The figure shows three views and two pictorial views of one solid part (mm, origin at its lowest corner). Answer the questions. A direction names the side the tool comes from. Coordinates: 2 decimals unless noted, no trailing zeros. Order: outer loops, then holes, each group sorted by start corner. A loop starts at its lowest first (then second) coordinate and runs counter-clockwise, first axis right, second up. Notation, with made-up numbers: (23.25, 66.5) -> (41.25, 66.5) arc R20 cw to (41.25, 93.5) -> close; hole circle Ø5 at (69.25, 56.25). An arc over 180 degrees is marked (long way). Write item = value, one per line.
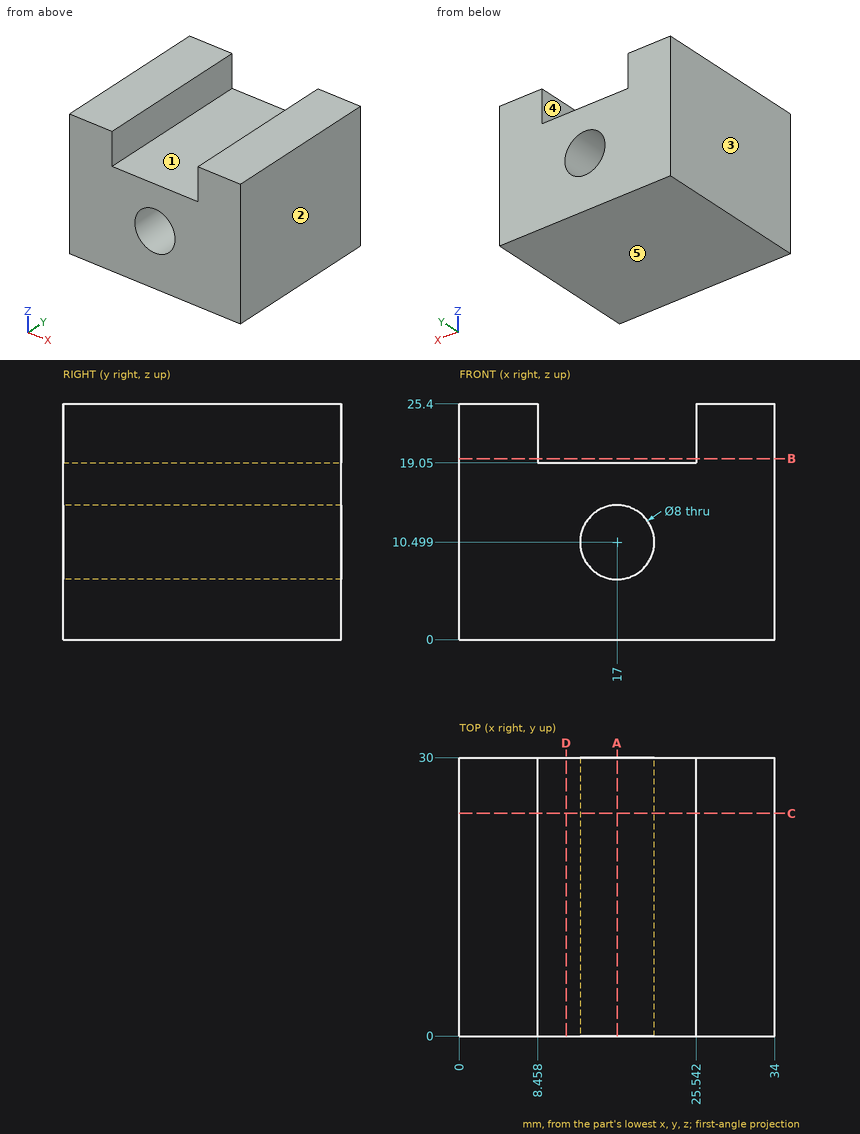
Q1. Section C-C, the plane y = 24 is taken. Give the vertices of the cut face in (x, z).
The answers:
outline = (0, 0) -> (34, 0) -> (34, 25.4) -> (25.54, 25.4) -> (25.54, 19.05) -> (8.46, 19.05) -> (8.46, 25.4) -> (0, 25.4) -> close; hole circle Ø8 at (17, 10.5)
Q2. The mould has two halves that part along X. Classify the marked faces 3, 4 and 5: released by +X, released by -X, zero draft, split by the parting line, or undercut.
The answers:
face_3 = released by -X
face_4 = undercut
face_5 = zero draft
Q3. Section A-A, the plane x = 17 is taken. Give the vertices of the cut face in (y, z).
The answers:
outline = (0, 0) -> (30, 0) -> (30, 6.5) -> (0, 6.5) -> close; (0, 14.5) -> (30, 14.5) -> (30, 19.05) -> (0, 19.05) -> close
Q4. Section D-D, the plane x = 11.5 is taken. Give the vertices of the cut face in (y, z), plus the area to 4 significant figures.
The answers:
outline = (0, 0) -> (30, 0) -> (30, 19.05) -> (0, 19.05) -> close
area = 571.5 mm2
Q5. Find the intervals of material crossed by line 1 along X through (y, z) = (17.5, 24.5); line 2 along Z through (x, y) = (17, 12.25); line 3 along X through (y, z) = (19.5, 10), in increasing order.
The answers:
line_1 = 0 to 8.46, 25.54 to 34
line_2 = 0 to 6.5, 14.5 to 19.05
line_3 = 0 to 13.03, 20.97 to 34
Q6. A tool of negligible diameter and unlimited length cuts with its end or side. For the marked faces 1 and 2, from which of +Z, -Z, +X, -X, +Y, -Y can it reach the whole face along a straight path? Write none if from no direction.
The answers:
face_1 = +Z, +Y, -Y
face_2 = +Z, -Z, +X, +Y, -Y
Q7. Section B-B, the plane z = 19.5 is taken. Give the vertices of the cut face in (x, y).
The answers:
outline = (0, 0) -> (8.46, 0) -> (8.46, 30) -> (0, 30) -> close; (25.54, 0) -> (34, 0) -> (34, 30) -> (25.54, 30) -> close
Q8. Each of these flat-tipped pins is pushed along its axis until it touches: pin 1 Ø7 at (y, z) = (13, 23) entering from -X; pin 2 Ø7 at (x, z) = (17, 10.5) entering from -Y; pin 3 Ø4 at (x, y) = (16, 12) entering from +Z. Where does it stop, or does it pass through?
The answers:
pin_1 = 0
pin_2 = through
pin_3 = 19.05
